from build123d import *

# Parameters (mm, degrees)
BOSS_EXTRUDE1_DEPTH = 12.7
SKETCH3_R           = 4
CUT_EXTRUDE1_DEPTH  = 50.99995
SKETCH4_R           = 4
CUT_EXTRUDE2_DEPTH  = 62.237182332


with BuildPart() as part:
    # Sketch2 → Boss-Extrude1 (new, symmetric)
    with BuildSketch(Plane.XY):
        with BuildLine():
            Line((-19.05, 0), (19.05, 0))
            Line((19.05, 0), (19.05, 50.8))
            Line((19.05, 50.8), (15.875, 50.8))
            ThreePointArc((15.875, 50.8), (13.62993597, 49.87006403), (12.7, 47.625))
            Line((12.7, 47.625), (12.7, 9.525))
            ThreePointArc((12.7, 9.525), (11.77006403, 7.27993597), (9.525, 6.35))
            Line((9.525, 6.35), (-15.875, 6.35))
            ThreePointArc((-15.875, 6.35), (-18.12006403, 5.42006403), (-19.05, 3.175))
            Line((-19.05, 3.175), (-19.05, 0))
        make_face()
    extrude(amount=BOSS_EXTRUDE1_DEPTH, both=True)

    # Sketch3 → Cut-Extrude1 (cut, through all)
    with BuildSketch(Plane(origin=(0, 6.35, 0), x_dir=(1, 0, 0), z_dir=(0, 1, 0))):
        with Locations(Location((-3.175, 0, 0), (0, 0, 180))):
            Circle(SKETCH3_R)
    extrude(amount=-CUT_EXTRUDE1_DEPTH, mode=Mode.SUBTRACT)

    # Sketch4 → Cut-Extrude2 (cut, through all)
    with BuildSketch(Plane.ZY.offset(-12.7)):
        with Locations(Location((0, 38.1, 0), (0, 0, 270))):
            Circle(SKETCH4_R)
        with Locations(Location((0, 19.05, 0), (0, 0, 90))):
            Circle(SKETCH4_R)
    extrude(amount=-CUT_EXTRUDE2_DEPTH, mode=Mode.SUBTRACT)


solid = part.part
Check sheet for the modelled part. Datum: model origin and axes. Units: mm. A direction names the side the tool comes from. Round coordinates to 2 decimals unless told otherwise and drop trailing zeros. Loops run counter-clockwise (first coordinate to the right, second up) from the corner with the lowest first, then second, coordinate; pieces in that order, holes last.
1. Scan lines: probe 1 along Z at (x, y) = (14, 19); probe 2 along Y at (x, z) = (15, 0.25); probe 3 along X at (y, z) = (40, 4.5). Record each from-to range of solid material in increasing order.
2. Gauge pin test, flat ends, axial feed: pin 1 Ø8 at (y, z) = (22, -1) entering from -X; pin 2 Ø2 at (x, z) = (3.5, -2.5) entering from +Y. Record the tip position at first contact, or that the pin passes through.
3. Mould release check, pull along Z, two halves, no side actions. Record for faces 3 (the flat face through (14, 16, -12.7)), 4 (the flat face through (17, 50.8, 0)), 5 (the cylindrical face through (0, 3.22, -2.43)): released by +Z, released by -Z, zero draft, split by the parting line, or undercut.
4. Sectioned sample at A-A on z = 0. Record the boundary of the cut face in (x, y) (3 decimals).
5. Sectioned sample at C-C on z = 10. Record the boundary of the cut face in (x, y) (3 decimals).
6. Set-up check for faces 1 (the flat face through (0, 6.35, 3)), 2 (the cylindrical face through (15.831, 15.876, 2.434)): record each of +Z, -Z, +X, -X, +Y, -Y from which the full face is reachable in a straight line by a thin tool's end or side.
7. Sectioned sample at B-B on y = 38.1. Record the boundary of the cut face in (x, z), and give its area (3 significant figures).
8. Sectioned sample at D-D on y = 44.5. Record the boundary of the cut face in (x, z).
Recorded:
1. probe 1: z = -12.7 to -4, 4 to 12.7
1. probe 2: y = 0 to 15.06, 23.04 to 34.11, 42.09 to 50.68
1. probe 3: x = 12.7 to 19.05
2. pin 1: stops at x = 12.7
2. pin 2: stops at y = 6.35
3. face 3: released by -Z
3. face 4: zero draft
3. face 5: undercut
4. outline: (-19.05, 0) - (-7.175, 0) - (-7.175, 6.35) - (-15.875, 6.35) arc R3.175 ccw to (-19.05, 3.175) - close; (0.825, 0) - (19.05, 0) - (19.05, 15.05) - (12.7, 15.05) - (12.7, 9.525) arc R3.175 cw to (9.525, 6.35) - (0.825, 6.35) - close; (12.7, 23.05) - (19.05, 23.05) - (19.05, 34.1) - (12.7, 34.1) - close; (12.7, 42.1) - (19.05, 42.1) - (19.05, 50.8) - (15.875, 50.8) arc R3.175 ccw to (12.7, 47.625) - close
5. outline: (-19.05, 0) - (19.05, 0) - (19.05, 50.8) - (15.875, 50.8) arc R3.175 ccw to (12.7, 47.625) - (12.7, 9.525) arc R3.175 cw to (9.525, 6.35) - (-15.875, 6.35) arc R3.175 ccw to (-19.05, 3.175) - close
6. face 1: +Z, -Z, -X, +Y
6. face 2: +X, -X
7. outline: (12.7, -12.7) - (19.05, -12.7) - (19.05, -4) - (12.7, -4) - close; (12.7, 4) - (19.05, 4) - (19.05, 12.7) - (12.7, 12.7) - close
7. area: 110 mm2
8. outline: (12.7, -12.7) - (19.05, -12.7) - (19.05, 12.7) - (12.7, 12.7) - close
